```python
from build123d import *

# Parameters (mm, degrees)
BOSS_EXTRUDE1_DEPTH             = 50
CHAMFER1_SIZE                   = 7
SKETCH2_R                       = 3.5
CUT_EXTRUDE1_DEPTH              = 62.524385409
SKETCH3_R                       = 1.75
CUT_EXTRUDE2_DEPTH              = 62.524385409
SKETCH5_R                       = 14
CUT_EXTRUDE4_DEPTH              = 3
BOSS_EXTRUDE2_DEPTH             = 7
CUT_EXTRUDE3_DEPTH              = 77.547867994
CUT_EXTRUDE3_DEPTH_BACK         = 77.547867994
SKETCH4_W                       = 51
SKETCH4_H                       = 47
SKETCH7_R                       = 1.25
SKETCH7_R_2                     = 5
CUT_EXTRUDE5_DEPTH              = 103.505990745
SKETCH8_R                       = 14.5
CUT_EXTRUDE6_DEPTH              = 3
SKETCH9_R                       = 3
CUT_EXTRUDE7_DEPTH              = 2
SKETCH11_R                      = 2
CUT_EXTRUDE8_DEPTH              = 10
BOSS_EXTRUDE3_START             = -32.5
BOSS_EXTRUDE3_DEPTH             = 65
SKETCH12_R                      = 2.6
CUT_EXTRUDE9_DEPTH              = 105.684053225
CUT_EXTRUDE10_DEPTH             = 3
BOSS_EXTRUDE4_DEPTH             = 3
SKETCH16_R                      = 1.75
CUT_EXTRUDE12_DEPTH             = 8
CHAMFER2_SIZE                   = 10
CUT_EXTRUDE14_DEPTH             = 10
CUT_EXTRUDE15_DEPTH             = 89.260982281
CUT_EXTRUDE15_DEPTH_BACK        = 89.260982281
CUT_EXTRUDE16_REACH             = 90.261
SKETCH19_R                      = 11
CUT_EXTRUDE16_DIRECTION_2_REACH = 90.261
CUT_EXTRUDE17_DEPTH             = 103.848193952


# Read off the part's stored shape, not the designer's step: Mirror1
with BuildPart() as part:
    # Sketch1 → Boss-Extrude1 (new body)
    with BuildSketch(Plane.XY):
        Polygon((-27.5, 0), (-27.5, 20), (0, 20), (0, 23), (-32.5, 23), (-32.5, 0), align=None)
    extrude(amount=BOSS_EXTRUDE1_DEPTH)

    # Chamfer1
    # the kernel refuses this chamfer: 7 mm, written as the material it takes off along each edge
    with BuildSketch(Plane(origin=(-32.5, 0, -18.001780916), x_dir=(-0.02749587661058612, 0.9996219169112968, 0), z_dir=(0, 0, 1))) as chamfer1_piece_1:
        Polygon((CHAMFER1_SIZE * 0.999621916911, -CHAMFER1_SIZE * 0.0274958766106), (-CHAMFER1_SIZE * 0.0274958766106, -CHAMFER1_SIZE * 0.999621916911), (0, 0), align=None)
    extrude(amount=86.003561832, mode=Mode.SUBTRACT)

    # Sketch2 → Cut-Extrude1 (cut, through all)
    with BuildSketch(Plane(origin=(-27.5, 0, 0), x_dir=(0, 0, -1), z_dir=(1, 0, 0))):
        with Locations((-35, 12)):
            Circle(SKETCH2_R)
    extrude(amount=-CUT_EXTRUDE1_DEPTH, mode=Mode.SUBTRACT)

    # Sketch3 → Cut-Extrude2 (cut, through all)
    with BuildSketch(Plane(origin=(-27.5, 0, 0), x_dir=(0, 0, -1), z_dir=(1, 0, 0))):
        with Locations((-10, 16)):
            Circle(SKETCH3_R)
        with Locations((-16, 16)):
            Circle(SKETCH3_R)
    extrude(amount=-CUT_EXTRUDE2_DEPTH, mode=Mode.SUBTRACT)

    # Sketch5 → Cut-Extrude4 (cut)
    with BuildSketch(Plane.ZY.offset(32.5)):
        with Locations((35, 12)):
            Circle(SKETCH5_R)
    extrude(amount=-CUT_EXTRUDE4_DEPTH, mode=Mode.SUBTRACT)

    # Sketch6 → Boss-Extrude2 (add)
    with BuildSketch(Plane.ZY.offset(32.5)):
        with BuildLine():
            Line((38.91656851, 42.559195759), (20, 23))
            Line((20, 23), (41.190648452, 23))
            ThreePointArc((41.190648452, 23), (45.305332833, 20.647646722), (50, 19.996268429))
            Line((50, 19.996268429), (50, 7))
            Line((50, 7), (61.474012963, 24.541456905))
            ThreePointArc((61.474012963, 24.541456905), (58.38884507, 43.808308659), (38.91656851, 42.559195759))
        make_face()
    extrude(amount=-BOSS_EXTRUDE2_DEPTH)

    # Mirror1: part across plane


with BuildPart() as part_1:
    add(part.part)
    add(part.part.mirror(Plane(origin=(0, 0, 0), x_dir=(0, 0, 1), z_dir=(1, 0, 0))))

    # Sketch4 → Cut-Extrude3 (cut, two sides: drawn at the far end of the back side and taken through both)
    with BuildSketch(Plane.XZ.offset(-20).offset(-CUT_EXTRUDE3_DEPTH_BACK)):
        with Locations((0, 26.5)):
            Rectangle(SKETCH4_W, SKETCH4_H)
    extrude(amount=CUT_EXTRUDE3_DEPTH + CUT_EXTRUDE3_DEPTH_BACK, mode=Mode.SUBTRACT)

    # Sketch7 → Cut-Extrude5 (cut, through all)
    with BuildSketch(Plane.ZY.offset(32.5)):
        with Locations(Location((41.557466488, 37.927777253, 0), (0, 0, 270))):
            Circle(SKETCH7_R)
        with Locations(Location((57.12135533, 27.029824962, 0), (0, 0, 270))):
            Circle(SKETCH7_R)
        with Locations(Location((47.6186816, 30.021344974, 0), (0, 0, 270))):
            Circle(SKETCH7_R_2)
    extrude(amount=-CUT_EXTRUDE5_DEPTH, mode=Mode.SUBTRACT)

    # Sketch8 → Cut-Extrude6 (cut)
    with BuildSketch(Plane.ZY.offset(32.5)):
        with Locations((47.6186816, 30.021344974)):
            Circle(SKETCH8_R)
    cut_extrude6 = extrude(amount=-CUT_EXTRUDE6_DEPTH, mode=Mode.SUBTRACT)

    # Sketch9 → Cut-Extrude7 (cut)
    with BuildSketch(Plane.ZY.offset(29.5)):
        with Locations(Location((41.557466488, 37.927777253, 0), (0, 0, 270))):
            Circle(SKETCH9_R)
        with Locations(Location((57.12135533, 27.029824962, 0), (0, 0, 270))):
            Circle(SKETCH9_R)
    cut_extrude7 = extrude(amount=-CUT_EXTRUDE7_DEPTH, mode=Mode.SUBTRACT)

    # Sketch11 → Cut-Extrude8 (cut)
    with BuildSketch(Plane(origin=(0, 0, 0), x_dir=(-1, 0, 0), z_dir=(0, 0, -1))):
        with Locations((-30, 15.523029521)):
            Circle(SKETCH11_R)
    cut_extrude8 = extrude(amount=-CUT_EXTRUDE8_DEPTH, mode=Mode.SUBTRACT)

    # Mirror2: Cut-Extrude6, Cut-Extrude7, Cut-Extrude8 across plane
    add(cut_extrude6.mirror(Plane(origin=(0, 0, 0), x_dir=(0, 0, 1), z_dir=(1, 0, 0))), mode=Mode.SUBTRACT)
    add(cut_extrude7.mirror(Plane(origin=(0, 0, 0), x_dir=(0, 0, 1), z_dir=(1, 0, 0))), mode=Mode.SUBTRACT)
    add(cut_extrude8.mirror(Plane(origin=(0, 0, 0), x_dir=(0, 0, 1), z_dir=(1, 0, 0))), mode=Mode.SUBTRACT)

    # Sketch10 → Boss-Extrude3 (add)
    with BuildSketch(Plane(origin=(0, 0, 0), x_dir=(0, 0, -1), z_dir=(1, 0, 0)).offset(BOSS_EXTRUDE3_START)):
        with BuildLine():
            Line((-38.91656851, 42.559195759), (-33.44256114, 36.899227268))
            ThreePointArc((-33.44256114, 36.899227268), (-53.026270805, 48.561620018), (-65.574367209, 29.533263138))
            Line((-65.574367209, 29.533263138), (-61.474012963, 24.541456905))
            ThreePointArc((-61.474012963, 24.541456905), (-58.38884507, 43.808308659), (-38.91656851, 42.559195759))
        make_face()
    extrude(amount=BOSS_EXTRUDE3_DEPTH)

    # Sketch12 → Cut-Extrude9 (cut, through all)
    with BuildSketch(Plane(origin=(32.5, 0, 0), x_dir=(0, 0, -1), z_dir=(1, 0, 0))):
        with Locations(Location((-10, 8, 0), (0, 0, 180))):
            Circle(SKETCH12_R)
    extrude(amount=-CUT_EXTRUDE9_DEPTH, mode=Mode.SUBTRACT)

    # Sketch13 → Cut-Extrude10 (cut)
    with BuildSketch(Plane(origin=(32.5, 0, 0), x_dir=(0, 0, -1), z_dir=(1, 0, 0))):
        with BuildLine():
            ThreePointArc((-13, 18.645751311), (-20, 16), (-13, 13.354248689))
            ThreePointArc((-13, 13.354248689), (-6, 16), (-13, 18.645751311))
        make_face()
    cut_extrude10 = extrude(amount=-CUT_EXTRUDE10_DEPTH, mode=Mode.SUBTRACT)

    # Mirror3: Cut-Extrude10 across plane
    add(cut_extrude10.mirror(Plane(origin=(0, 0, 0), x_dir=(0, 0, 1), z_dir=(1, 0, 0))), mode=Mode.SUBTRACT)

    # Sketch15 → Boss-Extrude4 (add)
    with BuildSketch(Plane(origin=(0, 0, 0), x_dir=(-1, 0, 0), z_dir=(0, 0, -1))):
        with BuildLine():
            Line((-14, 25), (-14, 23))
            Line((-14, 23), (-6, 23))
            Line((-6, 23), (-6, 25))
            ThreePointArc((-6, 25), (-10, 29), (-14, 25))
        make_face()
        with BuildLine():
            Line((6, 23), (6, 25))
            ThreePointArc((6, 25), (10, 29), (14, 25))
            Line((14, 25), (14, 23))
            Line((14, 23), (6, 23))
        make_face()
    extrude(amount=-BOSS_EXTRUDE4_DEPTH)

    # Sketch16 → Cut-Extrude12 (cut)
    with BuildSketch(Plane(origin=(0, 0, 0), x_dir=(-1, 0, 0), z_dir=(0, 0, -1))):
        with Locations((-10, 25)):
            Circle(SKETCH16_R)
        with Locations((10, 25)):
            Circle(SKETCH16_R)
    extrude(amount=-CUT_EXTRUDE12_DEPTH, mode=Mode.SUBTRACT)

    # Chamfer2
    chamfer2_edges = [part_1.edges().sort_by_distance(p)[0] for p in [
        (25.5, 21.5, 3),
        (-25.5, 21.5, 3),
    ]]
    chamfer(chamfer2_edges, length=CHAMFER2_SIZE)

    # Sketch17 → Cut-Extrude14 (cut)
    with BuildSketch(Plane(origin=(0, 0, 0), x_dir=(-1, 0, 0), z_dir=(0, 0, -1))):
        Polygon((-32.5, 18), (-32.5, 23), (-27.5, 23), align=None)
        Polygon((32.5, 23), (27.5, 23), (32.5, 18), align=None)
    extrude(amount=-CUT_EXTRUDE14_DEPTH, mode=Mode.SUBTRACT)

    # Sketch18 → Cut-Extrude15 (cut, two sides: drawn at the far end of the back side and taken through both)
    with BuildSketch(Plane(origin=(0, 0, 0), x_dir=(0, 0, -1), z_dir=(1, 0, 0)).offset(-CUT_EXTRUDE15_DEPTH_BACK)):
        with BuildLine():
            Line((-30.530550933, 2), (-50, 2))
            Line((-50, 2), (-58.261274719, 19.629826629))
            ThreePointArc((-58.261274719, 19.629826629), (-46.960735265, 6.780592155), (-30.530550933, 2))
        make_face()
    extrude(amount=CUT_EXTRUDE15_DEPTH + CUT_EXTRUDE15_DEPTH_BACK, mode=Mode.SUBTRACT)

    # Cut-Extrude16: up to this face of the body (flat: up to its plane)
    cut_extrude16_end = Plane(part_1.part.faces().sort_by_distance((-27.5, 11.293188811, 24.090581316))[0])
    # Sketch19 → Cut-Extrude16 (cut, up to the picked face)
    with BuildSketch(Plane(origin=(0, 0, 0), x_dir=(0, 0, -1), z_dir=(1, 0, 0)), mode=Mode.PRIVATE) as cut_extrude16_sk1:
        with Locations((-35, 12)):
            Circle(SKETCH19_R)
    cut_extrude16_tool1 = split(extrude(cut_extrude16_sk1.sketch, amount=-CUT_EXTRUDE16_REACH, mode=Mode.PRIVATE), bisect_by=cut_extrude16_end, keep=Keep.BOTH, mode=Mode.PRIVATE)
    add(cut_extrude16_tool1.solids().sort_by(Axis((0, 12, 35), (-1, 0, 0)))[0], mode=Mode.SUBTRACT)

    # Cut-Extrude16 direction 2: up to this face of the body (flat: up to its plane)
    cut_extrude16_direction_2_end = Plane(part_1.part.faces().sort_by_distance((27.5, 11.293188811, 24.090581316))[0])
    # Sketch19 → Cut-Extrude16 direction 2 (cut, up to the picked face)
    with BuildSketch(Plane(origin=(0, 0, 0), x_dir=(0, 0, -1), z_dir=(1, 0, 0)), mode=Mode.PRIVATE) as cut_extrude16_direction_2_sk1:
        with Locations((-35, 12)):
            Circle(SKETCH19_R)
    cut_extrude16_direction_2_tool1 = split(extrude(cut_extrude16_direction_2_sk1.sketch, amount=CUT_EXTRUDE16_DIRECTION_2_REACH, mode=Mode.PRIVATE), bisect_by=cut_extrude16_direction_2_end, keep=Keep.BOTH, mode=Mode.PRIVATE)
    add(cut_extrude16_direction_2_tool1.solids().sort_by(Axis((0, 12, 35), (1, 0, 0)))[0], mode=Mode.SUBTRACT)

    # Sketch20 → Cut-Extrude17 (cut, through all)
    with BuildSketch(Plane.ZY.offset(29.5)):
        with BuildLine():
            ThreePointArc((35.338857782, 16.153716102), (30.430818443, 15.855675228), (30.728859318, 10.947635889))
            ThreePointArc((30.728859318, 10.947635889), (33.235107626, 8.993143085), (35.965203237, 7.365905958))
            ThreePointArc((35.965203237, 7.365905958), (40.432511893, 9.479255027), (38.372112666, 13.971230754))
            ThreePointArc((38.372112666, 13.971230754), (36.800308025, 14.985787228), (35.338857782, 16.153716102))
        make_face()
    extrude(amount=-CUT_EXTRUDE17_DEPTH, mode=Mode.SUBTRACT)


solid = part_1.part
```
Verification items for the finished model (mm, model axes). A direction names the side the tool comes from. Give positions to 0.01 mm unless a question says otherwise; leave off trailing zeros. Write each loop counter-clockwise with the first axis right and the second up, starting at its lowest first coordinate (ties: lowest second). Pieces come first, ordered by that corner, then holes. Notation, with made-up numbers: (74, -5.5) - (96, -5.5) arc R25 cw to (96, 29.5) - close; hole circle Ø5 at (26.5, 59). An arc over 180 degrees is marked (long way). Put each result on its own line as item: value.
Q1. Depth check by flat-ended pin: P1, Ø6, axis at x = -2, y = 16, coming from the +Z side; P2, Ø3.5, axis at y = 27.03, z = 57.12, coming from the -X side; P3, Ø1.5, axis at x = -0.5, z = 1.5, coming from the +Y side; P4, Ø4, axis at y = 16, z = 10, coming from the +X side. Enter the tip coordinate at first touch or a pass-through.
Result:
P1: through
P2: x = -27.5
P3: y = 23
P4: x = 29.5
Q2. Section check A-A on x = 20. Record the cut outline in (y, z), and give its area (3 significant figures).
Result:
outline: (20, 0) - (23, 0) - (23, 7.5) - (20, 7.5) - close; (24.54, 61.47) arc R14.5 cw to (42.56, 38.92) - (36.9, 33.44) arc R16.5 ccw to (29.53, 65.57) - close
area: 117 mm2
Q3. Scan lines: probe 1 along X at (y, z) = (30, 59.5); probe 2 along Y at (x, z) = (-28.5, 16); probe 3 along X at (y, z) = (6.5, 34). Record each from-to range of solid material in increasing order. Write a range as from..to.
Result:
probe 1: -29.5..-25.5, 25.5..29.5
probe 2: 3..14.25, 17.75..23
probe 3: -29.5..-27.5, 27.5..29.5
Q4. Mould release check, pull along Y, two halves, no side actions. Record for faces 1 (the face through (0, 20, 2)), 2 (the face through (-26.51, 27.19, 58.36)), 3 (the face through (-14, 24, 1)): released by +Y, released by -Y, zero draft, split by the parting line, or undercut.
Result:
face 1: released by -Y
face 2: undercut
face 3: zero draft
Q5. Set-up check for faces 4 (the face through (-28.15, 14.76, 3.82)), 5 (the face through (-27.5, 38, 40)), 6 (the face through (-20.4, 21.5, 7.9)), 7 (the face through (-26, 20, 46)), 8 (the face through (-0.36, 39.77, 36.22)): record each of +Z, -Z, +X, -X, +Y, -Y from which the full face is reachable in a straight line by a thin tool's end or side.
Result:
face 4: -Z
face 5: -X
face 6: +Z, +Y, -Y
face 7: -Z, -Y
face 8: -Y
Q6. Section check C-C on z = 51.5. Record the cut outline in (x, y).
Result:
outline: (-32.5, 10.31) - (-25.5, 10.31) - (-25.5, 26.87) - (-29.5, 26.87) - (-29.5, 16.05) - (-32.5, 16.05) - close; (-32.5, 43.99) - (-29.5, 43.99) - (-29.5, 33.17) - (-25.5, 33.17) - (-25.5, 46.82) - (25.5, 46.82) - (25.5, 33.17) - (29.5, 33.17) - (29.5, 43.99) - (32.5, 43.99) - (32.5, 48.84) - (-32.5, 48.84) - close; (25.5, 10.31) - (32.5, 10.31) - (32.5, 16.05) - (29.5, 16.05) - (29.5, 26.87) - (25.5, 26.87) - close
Q7. Section check B-B on x = 10. Record the cut outline in (y, z), and give its area (3 significant figures).
Result:
outline: (20, 0) - (23.25, 0) - (23.25, 3) - (20, 3) - close; (24.54, 61.47) arc R14.5 cw to (42.56, 38.92) - (36.9, 33.44) arc R16.5 ccw to (29.53, 65.57) - close; (26.75, 0) - (29, 0) - (29, 3) - (26.75, 3) - close
area: 111 mm2
